Autodesk Inventor part; units mm, degrees
ref_plane "YZ Plane" through (0, 0, 0) normal (1, 0, 0) x (0, 1, 0)
ref_plane "XZ Plane" through (0, 0, 0) normal (0, 1, 0) x (-1, 0, 0)
ref_plane "XY Plane" through (0, 0, 0) normal (0, 0, 1) x (1, 0, 0)
sketch "Sketch1" plane through (0, 0, 0) normal (0, 0, 1) x (1, 0, 0)
  line L0 (6.35, 28.575) -> (25.4, 28.575)
  line L1 (6.35, 31.75) -> (25.4, 31.75)
  line L2 (25.4, 0) -> (6.35, 0)
  arc A0 (0, 6.35) -> (6.35, 0) centre (6.35, 6.35) ccw
  line L3 (0, 6.35) -> (0, 25.4)
  arc A1 (6.35, 31.75) -> (0, 25.4) centre (6.35, 25.4) ccw
  line L4 (6.35, 31.75) -> (25.4, 31.75)
  line L5 (25.4, 28.575) -> (6.35, 28.575)
  arc A2 (6.35, 28.575) -> (3.175, 25.4) centre (6.35, 25.4) ccw
  line L6 (3.175, 25.4) -> (3.175, 6.35)
  arc A3 (3.175, 6.35) -> (6.35, 3.175) centre (6.35, 6.35) ccw
  line L7 (6.35, 3.175) -> (25.4, 3.175)
  line L8 (28.575, 3.175) -> (28.575, 0)
  line L9 (25.4, 31.75) -> (28.575, 31.75)
  line L10 (28.575, 28.575) -> (25.4, 28.575)
  line L11 (28.575, 31.75) -> (28.575, 28.575)
  line L12 (28.575, 0) -> (25.4, 0)
  line L13 (28.575, 3.175) -> (28.575, 0)
  line L14 (25.4, 3.175) -> (28.575, 3.175)
  point P0 (0, 0)
extrude "Extrusion1" add sketch "Sketch1" against normal blind 584.2
chamfer "Chamfer1" distance 3.175 angle 45 4 edges at (28.575, 30.1625, 0) (28.575, 1.5875, 0) (28.575, 30.1625, -584.2) (28.575, 1.5875, -584.2)
sketch "Sketch2" plane through (6.35, 31.75, 0) normal (0, 1, 0) x (1, 0, 0)
  line L0 (19.05, 0) -> (0, 0)
  line L1 (22.225, 3.175) -> (22.225, 581.025)
  point P0 (-6.35, 0)
  point P1 (9.525, 12.7)
  dimension "d5" = 12.7
  dimension "d6" = 12.7
hole "Hole1" at (15.875, 31.75, -12.7) direction (0, -1, 0) diameter 6.7056 end through all
pattern_linear "Rectangular Pattern1" count 30 spacing 25.4 along (0, 0, -1) of "Hole1"
sketch "Sketch3" plane through (0, 6.35, 0) normal (-1, 0, 0) x (0, 0, 1)
  line L0 (0, 19.05) -> (-762, 19.05)
  line L1 (-762, 19.05) -> (-762, 0)
  line L2 (0, 0) -> (-762, 0)
  line L3 (0, 0) -> (0, 19.05)
  circle A0 centre (-701.3194, 9.525) radius 4.8006
  circle A1 centre (-111.4298, 9.525) radius 4.8006
  circle A2 centre (-189.2808, 9.525) radius 3.683
  circle A3 centre (-278.1808, 9.525) radius 3.683
  circle A4 centre (-483.7938, 9.525) radius 3.683
  circle A5 centre (-572.6938, 9.525) radius 3.683
  circle A6 centre (-471.1065, 9.525) radius 3.683
  circle A7 centre (-585.4065, 9.525) radius 3.683
  circle A8 centre (-290.8935, 9.525) radius 3.683
  circle A9 centre (-176.5935, 9.525) radius 3.683
  circle A10 centre (-553.7327, 9.525) radius 4.8006
  circle A11 centre (-528.3327, 9.525) radius 4.8006
  circle A12 centre (-502.9327, 9.525) radius 4.8006
  circle A13 centre (-259.0673, 9.525) radius 4.8006
  circle A14 centre (-233.6673, 9.525) radius 4.8006
  circle A15 centre (-208.2673, 9.525) radius 4.8006
  circle A16 centre (-609.6, 9.525) radius 1.5875
  circle A17 centre (-152.4, 9.525) radius 1.5875
  circle A18 centre (-381, 5.969) radius 4.8006
  circle A19 centre (-86.0298, 9.525) radius 4.8006
  circle A20 centre (-675.9194, 9.525) radius 4.8006
  circle A21 centre (-650.5194, 9.525) radius 4.8006
  circle A22 centre (-60.6298, 9.525) radius 4.8006
  point P0 (0, -6.35)
  point P1 (-762, -6.35)
extrude "Extrusion2" cut sketch "Sketch3" against normal up to next contours A0 | A1 | A2 | A3 | A4 | A5 | A6 | A7 | A8 | A9 | A10 | A11 | A12 | A13 | A14 | A15 | A16 | A17 | A18 | A19 | A20 | A21 | A22
properties part number "DBK_C-Channel_am-2222-23" material "Aluminum 6061"
CAD build for the part. Positions are in the model's coordinates, mm. A direction names the side the tool comes from. Give positions to 0.01 mm unless a question says otherwise; leave off trailing zeros. Return JSON: item names as keys, results as strings. Group by question number.
(1) Flat gauge pin, fed straight in: pin 1 Ø6 at (y, z) = (9, -481) entering from +X. Where does the tip first touch, or does it go through?
(2) Drill centre lines: L1, parallel to Y at x = 7.75, z = -545.5 (3 decimals); L2, parallel to X at y = 6.5, z = -34.5 (3 decimals); L3, parallel to Y at x = 1.5, z = -377. Where is each one in solid material? Low to high. Write a range as [from, to].
(3) 3-axis set-ups, long thin cutter, end or side, ignore diameter. For faces 4 (the face through (1.57, 17.32, -56.05)), 5 (the face through (17, 28.575, -288)): which of +Z, -Z, +X, -X, +Y, -Y reach the whole face in a straight line?
(4) Mould opens along Z. For faces 1 (the face through (0, 12, -288)), 2 (the face through (2, 12, 0)), 3 (the face through (1.565, 12.53, -385.796)) say: pulls with the +Z half, pulls with the -Z half, needs draft (parallel to the pull), parting line crosses it, or undercut.
Entries:
{
 "1": {"pin 1": "stops at x = 3.19"},
 "2": {"L1": "y = [0, 3.175], [28.575, 31.75]", "L2": "x = [0, 3.175]", "L3": "y = [2.25, 9.66], [14.97, 29.5]"},
 "3": {"face 4": "+X, -X", "face 5": "+Z, -Z, +X"},
 "4": {"face 1": "needs draft", "face 2": "pulls with the +Z half", "face 3": "undercut"}
}
